from build123d import *

# Parameters (mm, degrees)
ESQUISSE1_W        = 105
ESQUISSE1_H        = 18
ESQUISSE1_R        = 1
ESQUISSE1_R_2      = 0.5
ESQUISSE1_R_3      = 0.7
ESQUISSE1_R_4      = 2
BOSS_EXTRU_5_DEPTH = 0.5
ESQUISSE11_W       = 105
ESQUISSE11_H       = 1
BOSS_EXTRU_7_DEPTH = 4


with BuildPart() as part:
    # Esquisse1 → Boss.-Extru.5 (new body)
    with BuildSketch(Plane.XY):
        with Locations((52.5, 9)):
            Rectangle(ESQUISSE1_W, ESQUISSE1_H)
        with Locations((26, 9)):
            Circle(ESQUISSE1_R, mode=Mode.SUBTRACT)
        with Locations((32, 15)):
            Circle(ESQUISSE1_R_2, mode=Mode.SUBTRACT)
        with Locations((32, 9)):
            Circle(ESQUISSE1_R_2, mode=Mode.SUBTRACT)
        with Locations((32, 3)):
            Circle(ESQUISSE1_R_2, mode=Mode.SUBTRACT)
        with Locations((40, 15)):
            Circle(ESQUISSE1_R_2, mode=Mode.SUBTRACT)
        with Locations((40, 9)):
            Circle(ESQUISSE1_R_2, mode=Mode.SUBTRACT)
        with Locations((40, 3)):
            Circle(ESQUISSE1_R_2, mode=Mode.SUBTRACT)
        with Locations((44, 6)):
            Circle(ESQUISSE1_R_2, mode=Mode.SUBTRACT)
        with Locations((44, 12)):
            Circle(ESQUISSE1_R_2, mode=Mode.SUBTRACT)
        with Locations((48, 3)):
            Circle(ESQUISSE1_R_3, mode=Mode.SUBTRACT)
        with Locations((48, 9)):
            Circle(ESQUISSE1_R_3, mode=Mode.SUBTRACT)
        with Locations((48, 15)):
            Circle(ESQUISSE1_R_2, mode=Mode.SUBTRACT)
        with Locations((52.5, 6)):
            Circle(ESQUISSE1_R_4, mode=Mode.SUBTRACT)
        with Locations(Location((57, 15, 0), (0, 0, 180))):
            Circle(ESQUISSE1_R_2, mode=Mode.SUBTRACT)
        with Locations(Location((57, 9, 0), (0, 0, 180))):
            Circle(ESQUISSE1_R_3, mode=Mode.SUBTRACT)
        with Locations(Location((57, 3, 0), (0, 0, 180))):
            Circle(ESQUISSE1_R_3, mode=Mode.SUBTRACT)
        with Locations(Location((61, 12, 0), (0, 0, 180))):
            Circle(ESQUISSE1_R_2, mode=Mode.SUBTRACT)
        with Locations(Location((61, 6, 0), (0, 0, 180))):
            Circle(ESQUISSE1_R_2, mode=Mode.SUBTRACT)
        with Locations(Location((65, 3, 0), (0, 0, 180))):
            Circle(ESQUISSE1_R_2, mode=Mode.SUBTRACT)
        with Locations(Location((65, 9, 0), (0, 0, 180))):
            Circle(ESQUISSE1_R_2, mode=Mode.SUBTRACT)
        with Locations(Location((65, 15, 0), (0, 0, 180))):
            Circle(ESQUISSE1_R_2, mode=Mode.SUBTRACT)
        with Locations(Location((73, 3, 0), (0, 0, 180))):
            Circle(ESQUISSE1_R_2, mode=Mode.SUBTRACT)
        with Locations(Location((73, 9, 0), (0, 0, 180))):
            Circle(ESQUISSE1_R_2, mode=Mode.SUBTRACT)
        with Locations(Location((73, 15, 0), (0, 0, 180))):
            Circle(ESQUISSE1_R_2, mode=Mode.SUBTRACT)
        with Locations(Location((79, 9, 0), (0, 0, 180))):
            Circle(ESQUISSE1_R, mode=Mode.SUBTRACT)
    boss_extru_5 = extrude(amount=BOSS_EXTRU_5_DEPTH)

    # Esquisse11 → Boss.-Extru.7 (add)
    with BuildSketch(Plane.XY.offset(0.5)):
        with Locations((52.5, 0.5)):
            Rectangle(ESQUISSE11_W, ESQUISSE11_H)
        with Locations((52.5, 17.5)):
            Rectangle(ESQUISSE11_W, ESQUISSE11_H)
    boss_extru_7 = extrude(amount=BOSS_EXTRU_7_DEPTH)

    # Symétrie1: Boss.-Extru.5, Boss.-Extru.7 across plane
    add(boss_extru_5.mirror(Plane(origin=(0, 0, 0), x_dir=(1, 0, 0), z_dir=(0, 0, -1))))
    add(boss_extru_7.mirror(Plane(origin=(0, 0, 0), x_dir=(1, 0, 0), z_dir=(0, 0, -1))))


solid = part.part
Design review of the part built by this model. Coordinates are the model's own, in mm. A direction names the side the tool comes from. Give positions to 0.01 mm unless a question says otherwise; leave off trailing zeros. Loops run counter-clockwise (first coordinate to the right, second up) from the corner with the lowest first, then second, coordinate; pieces in that order, holes last. Notation, with made-up numbers: M 35,84 L 65,84 A20 cw 65,121 Z; hole C 28,87 d4. An arc over 180 degrees is marked long. One line per question, with ' | ' between items. Start each with the question number.
1. Insertion check: P1, Ø2, axis at x = 57, y = 9, coming from the -Z side; P2, Ø1.5, axis at x = 78.5, y = 14, coming from the +Z side; P3, Ø0.8, axis at x = 48, y = 3, coming from the +Z side. Each pin has a flat end and moves straight along its axis. Give the tip position at first contact, or say it passes through.
2. Add section A-A (x = 26). Write out the cut boundary in (y, z), plus the area to 3 significant figures.
3. To check wall thickness, follow L1, parallel to Y at x = 73, z = -0.15; L2, parallel to Y at x = 79, z = 0; L3, parallel to Y at x = 74, z = 3. State the ranges of each line that lie inside material, in increasing order.
4. For faces 1 (the face through (51.026, 7.352, -0.007)), 2 (the face through (52, 1, -2)), 3 (the face through (52, 9, 0.5)), list the 3-axis set-ups (+Z, -Z, +X, -X, +Y, -Y) from which the entire face can be reached by the end or side of a thin tool; tool diameter is ignored.
5. Add section D-D (y = 13.5). Write out the cut boundary in (x, z), plus the area to 3 significant figures.
6. Add section B-B (z = 3). Write out the cut boundary in (x, y).
7. Add section C-C (x = 15). Write out the cut boundary in (y, z).
8. The part is to be moulded in two halves that separate along X. For faces 4 (the face through (105, 8, 0)), 5 (the face through (52, 17, 2)), 6 (the face through (26, 10, 0)), say which applies: released by +X, released by -X, zero draft, split by the parting line, or undercut.
Worked out:
1) P1: stops at z = -0.5 | P2: stops at z = 0.5 | P3: passes through
2) outline: M 0,-4.5 L 1,-4.5 L 1,-0.5 L 8,-0.5 L 8,0.5 L 1,0.5 L 1,4.5 L 0,4.5 Z; M 10,-0.5 L 17,-0.5 L 17,-4.5 L 18,-4.5 L 18,4.5 L 17,4.5 L 17,0.5 L 10,0.5 Z | area: 32.0 mm²
3) L1: y = 0 to 2.5, 3.5 to 8.5, 9.5 to 14.5, 15.5 to 18 | L2: y = 0 to 8, 10 to 18 | L3: y = 0 to 1, 17 to 18
4) face 1: +Z, -Z | face 2: -Z, +X, -X | face 3: +Z, +X, -X
5) outline: M 0,-0.5 L 105,-0.5 L 105,0.5 L 0,0.5 Z | area: 105 mm²
6) outline: M 0,0 L 105,0 L 105,1 L 0,1 Z; M 0,17 L 105,17 L 105,18 L 0,18 Z
7) outline: M 0,-4.5 L 1,-4.5 L 1,-0.5 L 17,-0.5 L 17,-4.5 L 18,-4.5 L 18,4.5 L 17,4.5 L 17,0.5 L 1,0.5 L 1,4.5 L 0,4.5 Z
8) face 4: released by +X | face 5: zero draft | face 6: undercut
